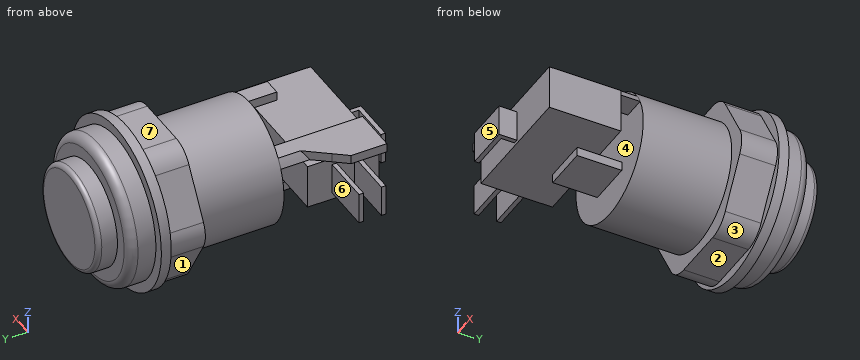
from build123d import *

# Parameters (mm, degrees)
CROQUIS1_R               = 11.5
SALIENTE_EXTRUIR1_DEPTH  = 4.5
REDONDEO1_R              = 1
CROQUIS2_R               = 16.25
SALIENTE_EXTRUIR2_DEPTH  = 6
REDONDEO2_R              = 2
CROQUIS3_R               = 13.75
SALIENTE_EXTRUIR3_DEPTH  = 30
CROQUIS5_R               = 18.5
SALIENTE_EXTRUIR4_DEPTH  = 2.2
SALIENTE_EXTRUIR5_DEPTH  = 8
REDONDEO3_R              = 6
CROQUIS7_W               = 10
CROQUIS7_H               = 2
SALIENTE_EXTRUIR6_DEPTH  = 10
CROQUIS8_W               = 10
CROQUIS8_H               = 2
SALIENTE_EXTRUIR7_DEPTH  = 11
SALIENTE_EXTRUIR8_DEPTH  = 2
CORTAR_EXTRUIR1_DEPTH    = 66.424097243
CROQUIS12_W              = 28
CROQUIS12_H              = 10
SALIENTE_EXTRUIR9_DEPTH  = 16
CROQUIS13_W              = 1
CROQUIS13_H              = 7
SALIENTE_EXTRUIR10_DEPTH = 4
CROQUIS14_W              = 7
CROQUIS14_H              = 1
SALIENTE_EXTRUIR11_DEPTH = 9
CROQUIS15_W              = 7
CROQUIS15_H              = 1
SALIENTE_EXTRUIR12_DEPTH = 11


with BuildPart() as part:
    # Croquis1 → Saliente-Extruir1 (new body)
    with BuildSketch(Plane(origin=(0, 0, 0), x_dir=(1, 0, 0), z_dir=(0, 1, 0))):
        with Locations(Location((0, 0, 0), (0, 0, 270))):
            Circle(CROQUIS1_R)
    extrude(amount=SALIENTE_EXTRUIR1_DEPTH)

    # Redondeo1
    redondeo1_edges = [part.edges().sort_by_distance(p)[0] for p in [
        (0, 4.5, -11.5),
    ]]
    fillet(redondeo1_edges, radius=REDONDEO1_R)

    # Croquis2 → Saliente-Extruir2 (add)
    with BuildSketch(Plane.XZ):
        with Locations(Location((0, 0, 0), (0, 0, 270))):
            Circle(CROQUIS2_R)
    extrude(amount=SALIENTE_EXTRUIR2_DEPTH)

    # Redondeo2
    redondeo2_edges = [part.edges().sort_by_distance(p)[0] for p in [
        (0, 0, 16.25),
    ]]
    fillet(redondeo2_edges, radius=REDONDEO2_R)

    # Croquis3 → Saliente-Extruir3 (add)
    with BuildSketch(Plane.XZ.offset(6)):
        with Locations(Location((0, 0, 0), (0, 0, 270))):
            Circle(CROQUIS3_R)
    extrude(amount=SALIENTE_EXTRUIR3_DEPTH)

    # Croquis5 → Saliente-Extruir4 (add)
    with BuildSketch(Plane.XZ.offset(6)):
        with Locations(Location((0, 0, 0), (0, 0, 270))):
            Circle(CROQUIS5_R)
    extrude(amount=SALIENTE_EXTRUIR4_DEPTH)

    # Croquis6 → Saliente-Extruir5 (add)
    with BuildSketch(Plane.XZ.offset(8.2)):
        Polygon((18.763883749, 0), (9.381941874, 16.25), (-9.381941874, 16.25), (-18.763883749, 0), (-9.381941874, -16.25), (9.381941874, -16.25), align=None)
    extrude(amount=SALIENTE_EXTRUIR5_DEPTH)

    # Redondeo3
    # the kernel refuses this fillet: 6 mm, written as the material it takes off along each edge
    with BuildSketch(Plane(origin=(9.381941874, -8.2, -16.25), x_dir=(-1, 0, 0), z_dir=(0, -1, 0))) as redondeo3_piece_1:
        with BuildLine():
            CenterArc((REDONDEO3_R * 0.57735026919, -REDONDEO3_R), REDONDEO3_R, 90, 60)
            Line((-REDONDEO3_R * 0.288675134595, -REDONDEO3_R * 0.5), (0, 0))
            Line((0, 0), (REDONDEO3_R * 0.57735026919, 0))
        make_face()
    extrude(amount=16.660254038, mode=Mode.SUBTRACT)
    with BuildSketch(Plane(origin=(18.763883749, -8.2, 0), x_dir=(-0.4999999999999997, 0, 0.8660254037844387), z_dir=(0, -1, 0)), Plane(origin=(9.381941874, -8.2, 16.25), x_dir=(-1, 0, 0), z_dir=(0, -1, 0)), Plane(origin=(-9.381941874, -8.2, 16.25), x_dir=(-0.5, 0, -0.8660254037844386), z_dir=(0, -1, 0)), Plane(origin=(-18.763883749, -8.2, 0), x_dir=(0.4999999999999992, 0, -0.866025403784439), z_dir=(0, -1, 0)), Plane(origin=(-9.381941874, -8.2, -16.25), x_dir=(1, 0, 0), z_dir=(0, -1, 0))) as redondeo3_piece_2:
        with BuildLine():
            CenterArc((REDONDEO3_R * 0.57735026919, REDONDEO3_R), REDONDEO3_R, 210, 60)
            Line((-REDONDEO3_R * 0.288675134595, REDONDEO3_R * 0.5), (0, 0))
            Line((0, 0), (REDONDEO3_R * 0.57735026919, 0))
        make_face()
    extrude(amount=16.660254038, mode=Mode.SUBTRACT)

    # Croquis7 → Saliente-Extruir6 (add)
    with BuildSketch(Plane.XZ.offset(36)):
        with BuildLine():
            Line((-7.489995997, 5.75), (-12.489995997, 5.75))
            ThreePointArc((-12.489995997, 5.75), (-11.965765437, 6.773696), (-11.357816692, 7.75))
            Line((-11.357816692, 7.75), (-7.489995997, 7.75))
            Line((-7.489995997, 7.75), (-7.489995997, 5.75))
        make_face()
        with BuildLine():
            Line((7.489995997, 7.75), (11.357816692, 7.75))
            ThreePointArc((11.357816692, 7.75), (11.965765437, 6.773696), (12.489995997, 5.75))
            Line((12.489995997, 5.75), (7.489995997, 5.75))
            Line((7.489995997, 5.75), (7.489995997, 7.75))
        make_face()
        with Locations((0, -5.25)):
            Rectangle(CROQUIS7_W, CROQUIS7_H)
    extrude(amount=SALIENTE_EXTRUIR6_DEPTH)

    # Croquis8 → Saliente-Extruir7 (add)
    with BuildSketch(Plane.XZ.offset(46)):
        with Locations((-12.489995997, 6.75)):
            Rectangle(CROQUIS8_W, CROQUIS8_H)
    extrude(amount=SALIENTE_EXTRUIR7_DEPTH)

    # Croquis9 → Saliente-Extruir8 (add)
    with BuildSketch(Plane.XY.offset(7.75)):
        Polygon((-17.489995997, -49), (-11.357816692, -41), (-11.357816692, -49), align=None)
    extrude(amount=-SALIENTE_EXTRUIR8_DEPTH)

    # Croquis11 → Cortar-Extruir1 (cut, through all)
    with BuildSketch(Plane.XY.offset(7.75)):
        Polygon((-15.190428757, -46), (-17.489995997, -49), (-17.489995997, -46), align=None)
    extrude(amount=-CORTAR_EXTRUIR1_DEPTH, mode=Mode.SUBTRACT)

    # Croquis12 → Saliente-Extruir9 (add)
    with BuildSketch(Plane(origin=(0, -41, 0), x_dir=(-1, 0, 0), z_dir=(0, -1, 0))):
        with Locations((0.25, -0.75)):
            Rectangle(CROQUIS12_W, CROQUIS12_H)
    extrude(amount=SALIENTE_EXTRUIR9_DEPTH)

    # Croquis13 → Saliente-Extruir10 (add)
    with BuildSketch(Plane.XZ.offset(57)):
        Rectangle(CROQUIS13_W, CROQUIS13_H)
    extrude(amount=SALIENTE_EXTRUIR10_DEPTH)

    # Croquis14 → Saliente-Extruir11 (add)
    with BuildSketch(Plane.ZY.offset(0.5)):
        with Locations((0, -60.5)):
            Rectangle(CROQUIS14_W, CROQUIS14_H)
    extrude(amount=SALIENTE_EXTRUIR11_DEPTH)

    # Croquis15 → Saliente-Extruir12 (add)
    with BuildSketch(Plane.ZY.offset(14.25)):
        with Locations((0.75, -47)):
            Rectangle(CROQUIS15_W, CROQUIS15_H)
        with Locations((0.75, -52)):
            Rectangle(CROQUIS15_W, CROQUIS15_H)
    extrude(amount=SALIENTE_EXTRUIR12_DEPTH)


solid = part.part
Can you work these out from the model? Positions are in its coordinate system, mm. Face numbers are marked on the shaded views. A direction names the side the tool comes from. Give positions to 0.01 mm unless a question says otherwise; leave off trailing zeros. Order: outer loops, then holes, each group sorted by start corner. A loop starts at its lowest first (then second) coordinate and runs counter-clockwise, first axis right, second up. Notation, with made-up numbers: M 88,0.25 L 105,0.25 A16 ccw 105,13.25 Z; hole C -2.5,67 d6. An arc over 180 degrees is marked long. Use one line per item in the form item = value. Start each with the question number.
Item 1: Will these pins go through, and if not, where does the flat tip stop? pin 1 Ø6.5 at (x, y) = (-1, -13.5) entering from -Z; pin 2 Ø1 at (x, z) = (1.5, -5.5) entering from -Y; pin 3 Ø5 at (y, z) = (-37, 14.5) entering from -X.
Item 2: If we section it at D-D (y = -3): Write out the boundary of the cut face in (x, z).
Item 3: If I drill on line 1 along Y through (x, z) = (-2, 2); line 2 along Y through (x, z) = (-21, 4); line 3 along Y through (x, z) = (-13, 12), over which ranges is the centre line in solid material (lowest first)?
Item 4: If we section it at C-C (y = -20.5): Write out the boundary of the cut face in (x, z), then the cut area to 3 significant figures.
Item 5: If we section it at A-A (x = -21): Write out the boundary of the cut face in (y, z), then the cut area to 3 significant figures.
Item 6: If we section it at B-B (y = -50.5): Write out the boundary of the cut face in (x, z), then the cut area to 3 significant figures.
Item 7: For the marked faces 1, 2 and 3, which set-ups out of +Z, -Z, +X, -X, +Y, -Y let a thin tool reach every point of the face, with its end or its side?
Item 8: We'd pull the mould along Y, two halves only. Please class the marked faces 4, 5, 6 and 7: +Y half, -Y half, draft (parallel to the pull), parting line (faces both ways), or undercut.
Outcome:
q1.pin_1 = -16.25
q1.pin_2 = -46
q1.pin_3 = -6.33
q2.outline = C 0,0 d32.5
q3.line_1 = -61 to -60, -57 to -41, -36 to 4.5
q3.line_2 = -52.5 to -51.5, -47.5 to -46.5
q3.line_3 = -8.2 to -6
q4.outline = C 0,0 d27.5
q4.area = 594 mm2
q5.outline = M -52.5,-2.75 L -51.5,-2.75 L -51.5,4.25 L -52.5,4.25 Z; M -47.5,-2.75 L -46.5,-2.75 L -46.5,4.25 L -47.5,4.25 Z
q5.area = 14.0 mm2
q6.outline = M -17.49,5.75 L -14.25,5.75 L -14.25,-4.25 L 13.75,-4.25 L 13.75,5.75 L -7.49,5.75 L -7.49,7.75 L -17.49,7.75 Z
q6.area = 300 mm2
q7.face_1 = -Z, -X, -Y
q7.face_2 = -Z, +X, -X, -Y
q7.face_3 = -Z, +X, -Y
q8.face_4 = undercut
q8.face_5 = -Y half
q8.face_6 = undercut
q8.face_7 = draft
